Geometry: final body of the model. Coordinates: model frame, mm. A direction names the side the tool comes from. Give positions to 0.01 mm unless a question says otherwise; leave off trailing zeros. Write each loop counter-clockwise with the first axis right and the second up, starting at its lowest first coordinate (ties: lowest second). Pieces come first, ordered by that corner, then holes.
Q1. Pin query (flat end, axial travel): pin 1 Ø4 at (x, y) = (1, -2.5) entering from -Z; pin 2 Ø2 at (x, z) = (0, 3) entering from +Y; pin 3 Ø0.5 at (y, z) = (-1, -1.5) entering from -X. Return the tip coordinate at first contact, or that it passes through.
Q2. Section A-A (x = 5.75). Return the cut outline in (y, z), plus the area to 3 significant figures.
Q3. Mould query, pull axis Z, two halves, no side actions, for faces 4 (the cylindrical face through (-2.218, 2.285, 3.584)), 5 (the flat face through (12, 0, 0)), 6 (the flat face through (-4, 0, -2)). Classes: +Z half, -Z half, draft (parallel to the pull), parting line (faces both ways), or undercut.
Q4. Line query: line 1 (X direction, y = -2.5, z = 2.75); line 2 (Z direction, x = -3.5, y = 2.25); line 3 (Z direction, x = -3, y = -1.5). Output: solid intervals per line, ascending.
Q5. Reachability of faces 1 (the flat face through (-3.768, -1.724, 1.014)), 2 (the flat face through (-5, 2, -2)), 3 (the flat face through (0, 2, -2)) from +Z, -Z, +X, -X, +Y, -Y: full face, straight path, thin tool, end or side. Return the list, or none.
Autodesk Inventor part; units mm, degrees
ref_plane "bolt_to_nut_XY" through (12, 0, 0) normal (1, 0, 0) x (0, 0, -1)
ref_plane "bolt_to_nut_YZ" through (12, 0, 0) normal (0, 0, -1) x (0, 1, 0)
ref_plane "bolt_to_nut_ZX" through (12, 0, 0) normal (0, 1, 0) x (1, 0, 0)
sketch "Sketch_1" plane through (0, 0, 0) normal (0, 0, 1) x (1, 0, 0)
  line L0 (12, 0) -> (-5, 0)
  line L1 (-5, 0) -> (-5, 3.75)
  line L2 (-5, 3.75) -> (-4.5, 4.25)
  line L3 (-4.5, 4.25) -> (0, 4.25)
  line L4 (0, 4.25) -> (0, 2.5)
  line L5 (0, 2.5) -> (11.5095, 2.5)
  line L6 (11.5095, 2.5) -> (12, 2.0095)
  line L7 (12, 2.0095) -> (12, 0)
  line L8 (12, 0) -> (-5, 0)
revolve "Revolution1" add sketch "Sketch_1" angle 360 about axis through (12, 0, 0) along (1, 0, 0)
thread "Thread1"
sketch "Sketch2" plane through (-5, 0, 0) normal (-1, 0, 0) x (0, 0, 1)
  point P0 (0, 0)
hole "Hole1" at (-5, 0, 0) direction (1, 0, 0) diameter 4 depth 2.5 tip angle 150
sketch "Sketch_3" plane through (-5, 0, 0) normal (1, 0, 0) x (0, 0, -1)
  line L0 (-2, 1.1547) -> (-2, -1.1547)
  line L1 (-2, -1.1547) -> (0, -2.3094)
  line L2 (0, -2.3094) -> (2, -1.1547)
  line L3 (2, -1.1547) -> (2, 1.1547)
  line L4 (2, 1.1547) -> (0, 2.3094)
  line L5 (0, 2.3094) -> (-2, 1.1547)
extrude "Extrusion1" cut sketch "Sketch_3" along normal blind 2.5
ref_plane "bolt_to_nut_XY" through (12, 0, 0) normal (1, 0, 0) x (0, 0, -1)
ref_plane "bolt_to_nut_YZ" through (12, 0, 0) normal (0, 0, -1) x (0, 1, 0)
ref_plane "bolt_to_nut_ZX" through (12, 0, 0) normal (0, 1, 0) x (1, 0, 0)
ref_plane "screw1_XY" through (0, 0, 0) normal (1, 0, 0) x (0, 0, -1)
ref_plane "screw1_YZ" through (0, 0, 0) normal (0, 0, -1) x (0, 1, 0)
ref_plane "screw1_ZX" through (0, 0, 0) normal (0, 1, 0) x (1, 0, 0)
properties part number "CB5-12" material "鋼、炭素鋼"
Computed:
1. pin 1: stops at z = -4.18
1. pin 2: stops at y = 3.75
1. pin 3: stops at x = -2.5
2. outline: circle Ø5 at (0, 0)
2. area: 19.6 mm2
3. face 4: parting line
3. face 5: draft
3. face 6: undercut
4. line 1: x = -5 to 0
4. line 2: z = -3.61 to -0.1, 0.1 to 3.61
4. line 3: z = -3.98 to -1.4, 1.4 to 3.98
5. face 1: -X
5. face 2: +Z, -Z, -X, +Y, -Y
5. face 3: +X
